from build123d import *

# Parameters (mm, degrees)
SKETCH1_W           = 48.26
SKETCH1_H           = 48.26
BOSS_EXTRUDE1_DEPTH = 1.016
FILLET1_R           = 15.24
BOSS_EXTRUDE2_DEPTH = 18.034
BOSS_EXTRUDE2_TAPER = 5
FILLET2_R           = 5.08


with BuildPart() as part:
    # Sketch1 → Boss-Extrude1 (new body)
    with BuildSketch(Plane(origin=(0, 19.05, 0), x_dir=(1, 0, 0), z_dir=(0, 1, 0))):
        Rectangle(SKETCH1_W, SKETCH1_H)
    extrude(amount=-BOSS_EXTRUDE1_DEPTH)

    # Fillet1
    fillet1_edges = [part.edges().sort_by_distance(p)[0] for p in [
        (-24.13, 18.542, -24.13),
        (24.13, 18.542, -24.13),
        (24.13, 18.542, 24.13),
        (-24.13, 18.542, 24.13),
    ]]
    fillet(fillet1_edges, radius=FILLET1_R)

    # Sketch2 → Boss-Extrude2 (add)
    with BuildSketch(Plane.XZ.offset(-18.034)):
        with BuildLine():
            Line((8.89, 20.066), (-8.89, 20.066))
            ThreePointArc((-8.89, 20.066), (-16.792625387, 16.792625387), (-20.066, 8.89))
            Line((-20.066, 8.89), (-20.066, -8.89))
            ThreePointArc((-20.066, -8.89), (-16.792625387, -16.792625387), (-8.89, -20.066))
            Line((-8.89, -20.066), (8.89, -20.066))
            ThreePointArc((8.89, -20.066), (16.792625387, -16.792625387), (20.066, -8.89))
            Line((20.066, -8.89), (20.066, 8.89))
            ThreePointArc((20.066, 8.89), (16.792625387, 16.792625387), (8.89, 20.066))
        make_face()
    extrude(amount=BOSS_EXTRUDE2_DEPTH, taper=BOSS_EXTRUDE2_TAPER)

    # Fillet2
    fillet2_edges = [part.edges().sort_by_distance(p)[0] for p in [
        (18.488229442, 0, 0),
        (15.676973126, 0, -15.676973126),
        (0, 0, -18.488229442),
        (-15.676973126, 0, -15.676973126),
        (-18.488229442, 0, 0),
        (-15.676973126, 0, 15.676973126),
        (0, 0, 18.488229442),
        (15.676973126, 0, 15.676973126),
    ]]
    fillet(fillet2_edges, radius=FILLET2_R)


solid = part.part
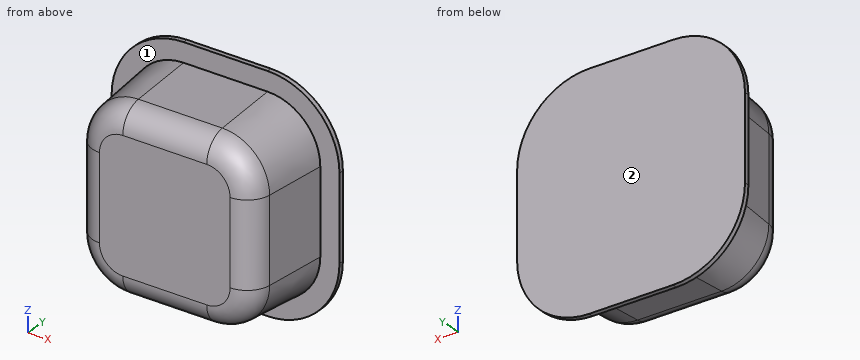
Source: CAD feature listing. Evaluate the final solid. Frame: model axes, mm. Face numbers are marked on the shaded views. A direction names the side the tool comes from. Round coordinates to 2 decimals unless told otherwise and drop trailing zeros. Answer as a JSON object with one key per item and string values. Group by question number.
Q1. Access query for the marked faces 1 and 2. Directions: +Z, -Z, +X, -X, +Y, -Y. A direction counts if a zero-diameter tool reaches every point of the face in a straight line with its end or side. Return the directions, or none.
Q2. Ray query, line 1 (X direction, y = 18, z = 5.5); line 2 (Z direction, x = 2, y = 4.75); line 3 (X direction, y = 17, z = -18). Return the intervals inside material, ascending. Write a range as from..to.
Q3. Contact query for flat-ended pins moving along their axis: P1, Ø1, axis at x = 18.5, y = 5, coming from the +Z side; P2, Ø8, axis at y = 4.5, z = -3, coming from the -X side; P3, Ø3, axis at y = 11, z = 8.5, coming from the +X side. Output: stop coordinate, or through.
Completed:
{
 "1": {"face 1": "-Y", "face 2": "+Z, -Z, +X, -X, +Y"},
 "2": {"line 1": "-20.06..20.06", "line 2": "-18.9..18.9", "line 3": "-15.21..15.21"},
 "3": {"P1": "z = 13.1", "P2": "x = -19.23", "P3": "x = 19.58"}
}
